For this review, use the dimensioned drawing (mm, ordinates from the lowest corner) and the shaded views. Give positions to 0.01 mm unless a question says otherwise; leave off trailing zeros. Order: outer loops, then holes, each group sorted by start corner. A loop starts at its lowest first (then second) coordinate and runs counter-clockwise, first axis right, second up.
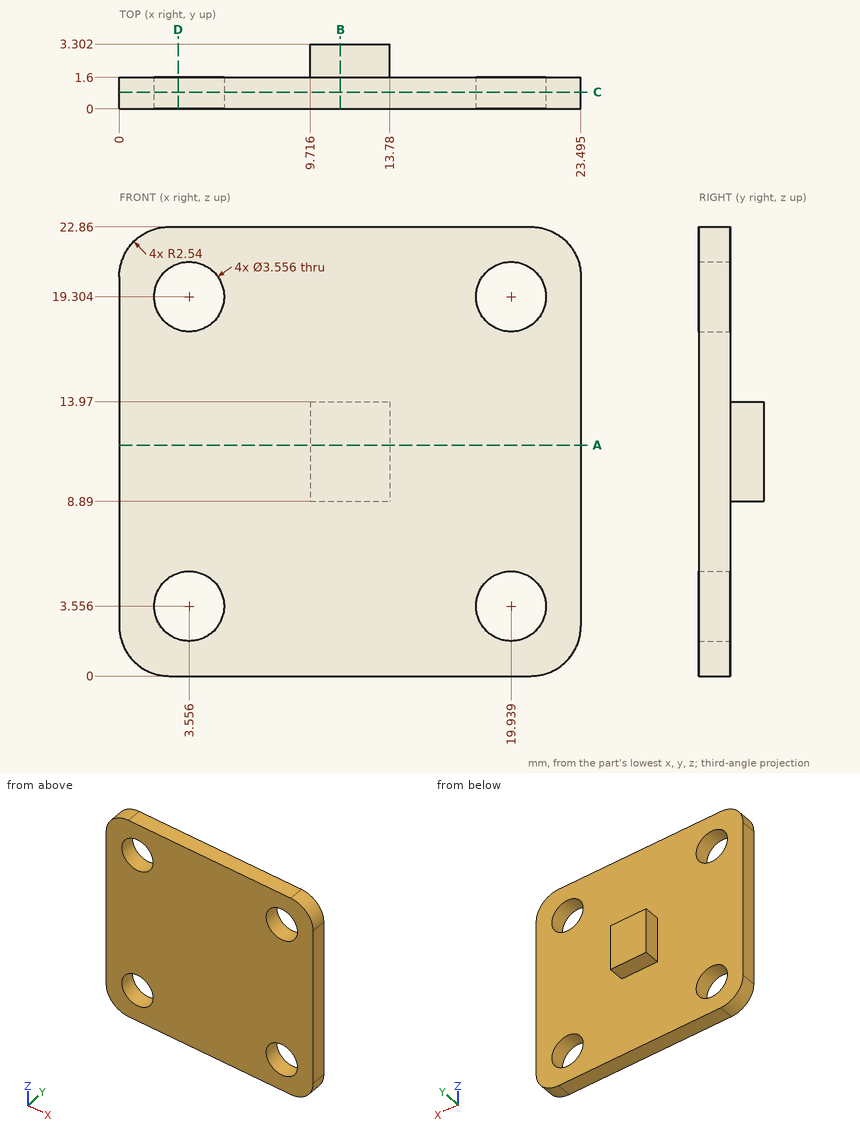
1. Take a section at A-A (z = 11.75). State the section outline as (x, y) points (1 decimal).
Recorded:
outline: (0, 0) - (23.5, 0) - (23.5, 1.6) - (13.8, 1.6) - (13.8, 3.3) - (9.7, 3.3) - (9.7, 1.6) - (0, 1.6) - close
2. For line 1 along Y through (x, z) = (16.5, 9); line 2 along X through (y, z) = (3, 9.25) (1 decimal); line 3 along X through (y, z) = (1, 20.5) (1 decimal), list the stretches that pass through material, from the lowest coordinate up.
Recorded:
line 1: y = 0 to 1.6
line 2: x = 9.7 to 13.8
line 3: x = 0 to 2.2, 4.9 to 18.6, 21.3 to 23.5
3. Take a section at C-C (y = 0.85). State the section outline as (x, z) points (1 decimal), then the cut area to 3 significant figures.
Recorded:
outline: (0, 2.5) arc R2.5 ccw to (2.5, 0) - (21, 0) arc R2.5 ccw to (23.5, 2.5) - (23.5, 20.3) arc R2.5 ccw to (21, 22.9) - (2.5, 22.9) arc R2.5 ccw to (0, 20.3) - close; hole circle Ø3.6 at (3.6, 3.6); hole circle Ø3.6 at (3.6, 19.3); hole circle Ø3.6 at (19.9, 3.6); hole circle Ø3.6 at (19.9, 19.3)
area: 492 mm2
4. For pin 1 (0.5 mm diameter, centred on x = 12.5, y = 2.5, fed in from -Z); pin 2 (0.5 mm diameter, centred on x = 11.5, y = 2, fed in from +Z); pin 3 (1.5 mm diameter, centred on x = 16, z = 2.5, fed in from +Y), all flat-tipped, find the tip position at first contact; note any pin that passes through.
Recorded:
pin 1: stops at z = 8.89
pin 2: stops at z = 13.97
pin 3: stops at y = 1.6
5. Take a section at B-B (x = 11.25). State the section outline as (y, z) points.
Recorded:
outline: (0, 0) - (1.6, 0) - (1.6, 8.89) - (3.3, 8.89) - (3.3, 13.97) - (1.6, 13.97) - (1.6, 22.86) - (0, 22.86) - close
6. Take a section at D-D (x = 3). State the section outline as (y, z) points (1 decimal).
Recorded:
outline: (0, 0) - (1.6, 0) - (1.6, 1.9) - (0, 1.9) - close; (0, 5.2) - (1.6, 5.2) - (1.6, 17.6) - (0, 17.6) - close; (0, 21) - (1.6, 21) - (1.6, 22.9) - (0, 22.9) - close
